Verification items for the finished model (mm, model axes). A direction names the side the tool comes from. Coordinates: 2 decimals unless noted, no trailing zeros. Loops run counter-clockwise (first coordinate to the right, second up) from the corner with the lowest first, then second, coordinate; pieces in that order, holes last. Notation, with made-up numbers: M 10,31.25 L 20,31.25 A20 ccw 20,43.25 Z; hole C -36.5,86 d4. An arc over 180 degrees is marked long. Write item = value, one per line. Start each with the question number.
```python
from build123d import *

# Parameters (mm, degrees)
SKETCH_1_R          = 35
SKETCH_1_R_2        = 22
EXTRUDE_1_DEPTH     = 3
SKETCH_2_R          = 35
SKETCH_2_R_2        = 23.75
EXTRUDE_2_DEPTH     = 14
SKETCH_4_R          = 2.15
CUT_EXTRUDE_1_DEPTH = 70
FILLET_1_R          = 2


with BuildPart() as part:
    # 草图1 → 凸台-拉伸1 (new body)
    with BuildSketch(Plane(origin=(0, 0, 0), x_dir=(1, 0, 0), z_dir=(0, 1, 0))):
        with Locations(Location((0, 0, 0), (0, 0, 270))):
            Circle(SKETCH_1_R)
        with Locations(Location((0, 0, 0), (0, 0, 270))):
            Circle(SKETCH_1_R_2, mode=Mode.SUBTRACT)
    extrude(amount=EXTRUDE_1_DEPTH)

    # 草图2 → 凸台-拉伸2 (add)
    with BuildSketch(Plane(origin=(0, 3, 0), x_dir=(1, 0, 0), z_dir=(0, 1, 0))):
        with Locations(Location((0, 0, 0), (0, 0, 270))):
            Circle(SKETCH_2_R)
        with Locations(Location((0, 0, 0), (0, 0, 270))):
            Circle(SKETCH_2_R_2, mode=Mode.SUBTRACT)
    extrude(amount=EXTRUDE_2_DEPTH)

    # 草图4 → 切除-拉伸1 (cut)
    with BuildSketch(Plane(origin=(0, 0, 0), x_dir=(1, 0, 0), z_dir=(0, 1, 0))):
        with Locations(Location((29, 0, 0), (0, 0, 270))):
            Circle(SKETCH_4_R)
        with Locations(Location((-14.5, -25.11473671, 0), (0, 0, 270))):
            Circle(SKETCH_4_R)
        with Locations(Location((-14.5, 25.11473671, 0), (0, 0, 270))):
            Circle(SKETCH_4_R)
    extrude(amount=CUT_EXTRUDE_1_DEPTH, mode=Mode.SUBTRACT)

    # 圆角1
    fillet_1_edges = [part.edges().sort_by_distance(p)[0] for p in [
        (29, 0, -2.15),
        (-14.5, 0, 22.96473671),
        (-14.5, 0, -27.26473671),
    ]]
    fillet(fillet_1_edges, radius=FILLET_1_R)


solid = part.part
```
Q1. Sectioned sample at B-B on z = 0. Record the cut outline in (x, y), plus the area to 3 significant figures.
Q2. Scan lines: L1, parallel to X at y = 8, z = 0; L2, parallel to X at y = 12, z = -1; L3, parallel to Z at x = -14.5, y = 8.75. Record each from-to range of solid material in increasing order. Write a range as [from, to].
Q3. Gauge pin test, flat ends, axial feed: pin 1 (2 mm diameter, centred on x = 16, z = -13, fed in from +Y); pin 2 (3 mm diameter, centred on x = 9, y = 2, fed in from -Z); pin 3 (5 mm diameter, centred on y = 2, z = 1.5, fed in from -X); pin 4 (7 mm diameter, centred on x = -14.5, z = 25.11, fed in from -Y). Record the tip position at first contact, or that the pin passes through.
Q4. Sectioned sample at C-C on y = 13.25. Record the cut outline in (x, z), plus the area to 3 significant figures.
Q5. Set-up check for faces 1 (the face through (-21.477, 1.479, -4.769)), 2 (the face through (-23.185, 9.902, -5.149)): record each of +Z, -Z, +X, -X, +Y, -Y from which the full face is reachable in a straight line by a thin tool's end or side.
Q6. Mould release check, pull along Z, two halves, no side actions. Record for faces 3 (the face through (-16, 3, 16)), 4 (the face through (-21, 8, -28)), 5 (the face through (-16.6, 9.4, 24.65)), 6 (the face through (-7, 17, 23)): +Z half, -Z half, draft (parallel to the pull), parting line (faces both ways), or undercut.
Q7. Sectioned sample at A-A on x = 0. Record the cut outline in (y, z), plus the area to 3 significant figures.
Q8. Sectioned sample at D-D on z = -16. Record the cut outline in (x, y).
Solutions:
q1.outline = M -35,0 L -22,0 L -22,3 L -23.75,3 L -23.75,17 L -35,17 Z; M 22,0 L 24.85,0 A2 ccw 26.85,2 L 26.85,17 L 23.75,17 L 23.75,3 L 22,3 Z; M 31.15,2 A2 ccw 33.15,0 L 35,0 L 35,17 L 31.15,17 Z
q1.area = 318 mm²
q2.L1 = [-35, -23.75], [23.75, 26.85], [31.15, 35]
q2.L2 = [-34.99, -23.73], [23.73, 27.1], [30.9, 34.99]
q2.L3 = [-31.86, -27.26], [-22.96, -18.81], [18.81, 22.96], [27.26, 31.86]
q3.pin_1 = through
q3.pin_2 = -34.19
q3.pin_3 = -35
q3.pin_4 = 0.11
q4.outline = C 0,0 d70; hole C 0,0 d47.5; hole C -14.5,-25.11 d4.3; hole C -14.5,25.11 d4.3; hole C 29,0 d4.3
q4.area = 2,030 mm²
q5.face_1 = +Y, -Y
q5.face_2 = +Y
q6.face_3 = undercut
q6.face_4 = parting line
q6.face_5 = undercut
q6.face_6 = draft
q7.outline = M 0,-35 L 17,-35 L 17,-23.75 L 3,-23.75 L 3,-22 L 0,-22 Z; M 0,22 L 3,22 L 3,23.75 L 17,23.75 L 17,35 L 0,35 Z
q7.area = 393 mm²
q8.outline = M -31.13,0 L -15.1,0 L -15.1,3 L -17.55,3 L -17.55,17 L -31.13,17 Z; M 15.1,0 L 31.13,0 L 31.13,17 L 17.55,17 L 17.55,3 L 15.1,3 Z
